```python
from build123d import *

# Parameters (mm, degrees)
F0_R           = 12.1
F0_R_2         = 3.925
F1_DEPTH       = 8
F2_D           = 5
F2_DEPTH       = 12
F2_CBORE_D     = 7
F2_CBORE_DEPTH = 9
F2_TIP         = 1.5021515476
F3_R           = 7


# Not quite as in the source:
# - a feature names something its author has since deleted; it is built from what else it names


with BuildPart() as f1:
    # F0 (on Top) → F1 (new body)
    with BuildSketch(Plane.XY):
        Circle(F0_R)
        with BuildLine():
            Line((-8.3705968588, -6.0454343887), (-7.2080156238, -4.737418765))
            ThreePointArc((-7.2080156238, -4.737418765), (-4.737418765, -4.5919843762), (-4.5919843762, -7.062581235))
            Line((-4.5919843762, -7.062581235), (-5.7545656113, -8.3705968588))
            ThreePointArc((-5.7545656113, -8.3705968588), (-8.22516247, -8.5160312475), (-8.3705968588, -6.0454343887))
        make_face(mode=Mode.SUBTRACT)
        with BuildLine():
            ThreePointArc((4.5919843762, -7.062581235), (4.737418765, -4.5919843762), (7.2080156238, -4.737418765))
            Line((7.2080156238, -4.737418765), (8.3705968588, -6.0454343887))
            ThreePointArc((8.3705968588, -6.0454343887), (8.22516247, -8.5160312475), (5.7545656113, -8.3705968588))
            Line((5.7545656113, -8.3705968588), (4.5919843762, -7.062581235))
        make_face(mode=Mode.SUBTRACT)
        with BuildLine():
            ThreePointArc((-8.3705968588, 6.0454343887), (-8.22516247, 8.5160312475), (-5.7545656113, 8.3705968588))
            Line((-5.7545656113, 8.3705968588), (-4.5919843762, 7.062581235))
            ThreePointArc((-4.5919843762, 7.062581235), (-4.737418765, 4.5919843762), (-7.2080156238, 4.737418765))
            Line((-7.2080156238, 4.737418765), (-8.3705968588, 6.0454343887))
        make_face(mode=Mode.SUBTRACT)
        Circle(F0_R_2, mode=Mode.SUBTRACT)
        with BuildLine():
            Line((8.3705968588, 6.0454343887), (7.2080156238, 4.737418765))
            ThreePointArc((7.2080156238, 4.737418765), (4.737418765, 4.5919843762), (4.5919843762, 7.062581235))
            Line((4.5919843762, 7.062581235), (5.7545656113, 8.3705968588))
            ThreePointArc((5.7545656113, 8.3705968588), (8.22516247, 8.5160312475), (8.3705968588, 6.0454343887))
        make_face(mode=Mode.SUBTRACT)
    extrude(amount=-F1_DEPTH)

    # F2
    with Locations(Plane.XY):
        with Locations((-5.9, 5.9), (-7.062581235, 7.2080156238), (-7.062581235, -7.2080156238), (7.062581235, -7.2080156238), (5.9, -5.9), (5.9, 5.9), (7.062581235, 7.2080156238), (-5.9, -5.9)):
            CounterBoreHole(F2_D / 2, F2_CBORE_D / 2, F2_CBORE_DEPTH, depth=F2_DEPTH)
            with Locations((0, 0, -(F2_DEPTH + F2_TIP / 2))):  # 118° drill point
                Cone(0, F2_D / 2, F2_TIP, mode=Mode.SUBTRACT)

    # F3
    f3_edges = [f1.edges().sort_by_distance(p)[0] for p in [
        (12.1, 0, -8),
        (0, 12.1, -8),
        (-12.1, 0, -8),
        (0, -12.1, -8),
    ]]
    fillet(f3_edges, radius=F3_R)


solid = f1.part
```
Can you work these out from the model? Positions are in its coordinate system, mm. A direction names the side the tool comes from. Round coordinates to 2 decimals unless told otherwise and drop trailing zeros. Return JSON: item names as keys, results as strings. Group by question number.
1. I need wall thicknesses on line 1 (Y direction, x = 3.5, z = -4.5); line 2 (Y direction, x = 4.25, z = -1.75); line 3 (Y direction, x = 5, z = -0.5). Which ranges of each line are inside material? Lowest first, please. Write a range as [from, to].
2. If we section it at A-A, the plane y = 5.75: Count the separate pieces of the cut face and the enclosed holes in it, then the cut area to 3 significant figures.
3. We'd pull the mould along X, two halves only. Please class faces 6 (the face through (4.551, -9.646, -2.413)), 7 (the face through (-0.1, -12.1, -0.5)), 8 (the face through (3.509, 3.344, -3.944)), 9 (the face through (-4.578, -9.673, -2.413)): released by +X, released by -X, zero draft, split by the parting line, or undercut.
4. Which directions (+Z, -Z, +X, -X, +Y, -Y) give clear straight access to the entire face, cutting with the end or side of a thin tool? Please do faces 1 (the face through (9.72, -4.93, -2.3)), 2 (the face through (-3.64, 3.23, -3.94)), 3 (the face through (-4.551, 9.646, -2.413)), 4 (the face through (9.694, 4.901, -2.295)), 5 (the face through (4.578, 9.673, -2.413)).
5. Will these pins go through, and if not, where does the flat tip stop? pin 1 (4 mm diameter, centred on y = 6.5, z = -4, fed in from +X); pin 2 (1.5 mm diameter, centred on x = -2.5, z = -6.5, fed in from -Y); pin 3 (2 mm diameter, centred on x = -3, z = -3.5, fed in from +Y).
Output values:
{
 "1": {"line 1": "[-10.6, -8.45], [-3.35, -1.78], [1.78, 3.35], [8.45, 10.6]", "line 2": "[-11.29, -9.29], [-2.81, 2.81], [9.29, 11.29]", "line 3": "[-11.02, -10.04], [-2.52, 2.52], [10.04, 11.02]"},
 "2": {"separate pieces": "3", "enclosed holes": "0", "area": "40.2 mm²"},
 "3": {"face 6": "released by +X", "face 7": "split by the parting line", "face 8": "undercut", "face 9": "released by -X"},
 "4": {"face 1": "+Z, -Z, -Y", "face 2": "+Z, -Z", "face 3": "+Z, -Z, -X", "face 4": "+Z, -Z, +Y", "face 5": "+Z, -Z, +X"},
 "5": {"pin 1": "x = 10.81", "pin 2": "y = -9.95", "pin 3": "y = 11.65"}
}
